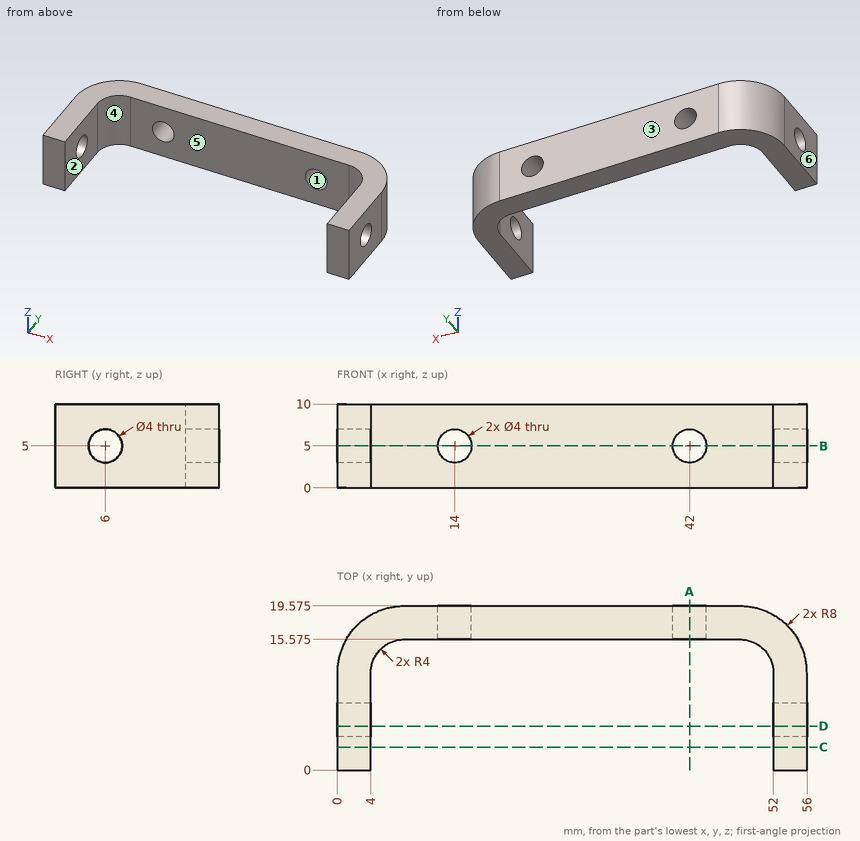
Study the drawing (mm; zero at the part's minimum x, y, z) and answer. A direction names the side the tool comes from. Round coordinates to 2 decimals unless told otherwise and drop trailing zeros. Write each loop counter-clockwise with the first axis right and the second up, starting at its lowest first coordinate (ties: lowest second). Pieces come first, ordered by that corner, then holes.
Q1. The mould has two halves that part along X. Classify the marked faces 3, 4, 5 and 6: released by +X, released by -X, zero draft, split by the parting line, or undercut.
Values:
face 3: zero draft
face 4: undercut
face 5: undercut
face 6: released by -X
Q2. Flat-ended cylindrical pins translate along their axes: P1, Ø1.5, axis at x = 31, y = 15.5, coming from the +Z side; P2, Ø3, axis at x = 42, z = 5, coming from the +Y side; P3, Ø4.5, axis at x = 14, z = 5, coming from the -Y side (3 decimals). Find the tip coordinate at first contact, or state that the pin passes through.
Values:
P1: stops at z = 10
P2: passes through
P3: stops at y = 15.575
Q3. Find section C-C on y = 2.75. Determine the outline of the cut face in (x, z).
Values:
outline: (0, 0) - (4, 0) - (4, 10) - (0, 10) - close; (52, 0) - (56, 0) - (56, 10) - (52, 10) - close
Q4. Find section D-D on y = 5.25. Determine the outline of the cut face in (x, z).
Values:
outline: (0, 0) - (4, 0) - (4, 3.15) - (0, 3.15) - close; (0, 6.85) - (4, 6.85) - (4, 10) - (0, 10) - close; (52, 0) - (56, 0) - (56, 3.15) - (52, 3.15) - close; (52, 6.85) - (56, 6.85) - (56, 10) - (52, 10) - close
Q5. A tool of negligible diameter and unlimited length cuts with its end or side. For the marked faces 1 and 2, from which of +Z, -Z, +X, -X, +Y, -Y can it reach the whole face along a straight path? Write none if from no direction.
Values:
face 1: +Y, -Y
face 2: +Z, -Z, -Y
Q6. Straight lines are drawn through the part: line 1 (Z direction, x = 1.85, y = 6); line 2 (X direction, y = 9.5, z = 8.75); line 3 (X direction, y = 18.15, z = 5). For each, find the intervals that lie inside material, in ascending order.
Values:
line 1: z = 0 to 3, 7 to 10
line 2: x = 0 to 4, 52 to 56
line 3: x = 3.44 to 12, 16 to 40, 44 to 52.56
Q7. Find section B-B on z = 5. Determine the outline of the cut face in (x, y) (1 decimal).
Values:
outline: (0, 0) - (4, 0) - (4, 4) - (0, 4) - close; (0, 8) - (4, 8) - (4, 11.6) arc R4 cw to (8, 15.6) - (12, 15.6) - (12, 19.6) - (8, 19.6) arc R8 ccw to (0, 11.6) - close; (16, 15.6) - (40, 15.6) - (40, 19.6) - (16, 19.6) - close; (44, 15.6) - (48, 15.6) arc R4 cw to (52, 11.6) - (52, 8) - (56, 8) - (56, 11.6) arc R8 ccw to (48, 19.6) - (44, 19.6) - close; (52, 0) - (56, 0) - (56, 4) - (52, 4) - close
Q8. Find section A-A on x = 42. Determine the outline of the cut face in (y, z) (1 decimal).
Values:
outline: (15.6, 0) - (19.6, 0) - (19.6, 3) - (15.6, 3) - close; (15.6, 7) - (19.6, 7) - (19.6, 10) - (15.6, 10) - close
